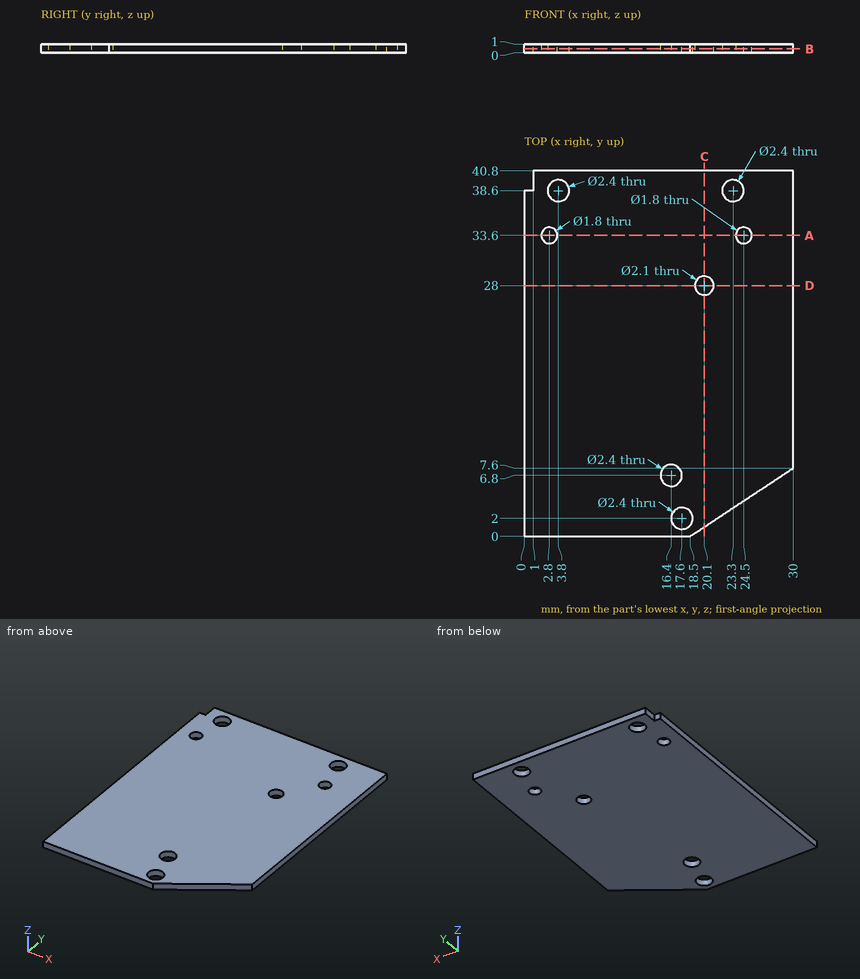
Source: three-view drawing plus pictorial views. Frame: mm from the lowest corner of the part. Coordinates: 2 decimals unless noted, no trailing zeros. Order: outer loops, then holes, each group sorted by start corner. A loop starts at its lowest first (then second) coordinate and runs counter-clockwise, first axis right, second up.
1) Section B-B (z = 0.45). Return loops of the section in (x, y), then the cut area to 3 significant figures.
Result sheet:
outline: (0, 0) - (18.5, 0) - (30, 7.6) - (30, 40.8) - (1, 40.8) - (1, 38.6) - (0, 38.6) - close; hole circle Ø1.8 at (2.8, 33.6); hole circle Ø2.4 at (3.8, 38.6); hole circle Ø2.4 at (16.4, 6.8); hole circle Ø2.4 at (17.6, 2); hole circle Ø2.1 at (20.1, 28); hole circle Ø2.4 at (23.3, 38.6); hole circle Ø1.8 at (24.5, 33.6)
area: 1,150 mm2
2) Section D-D (y = 28). Return loops of the section in (x, z).
Result sheet:
outline: (0, 0) - (19.05, 0) - (19.05, 1) - (0, 1) - close; (21.15, 0) - (30, 0) - (30, 1) - (21.15, 1) - close
3) Section A-A (y = 33.6). Return loops of the section in (x, z), then the cut area to 3 significant figures.
Result sheet:
outline: (0, 0) - (1.9, 0) - (1.9, 1) - (0, 1) - close; (3.7, 0) - (23.6, 0) - (23.6, 1) - (3.7, 1) - close; (25.4, 0) - (30, 0) - (30, 1) - (25.4, 1) - close
area: 26.4 mm2
4) Section C-C (x = 20.1). Return loops of the section in (y, z).
Result sheet:
outline: (1.06, 0) - (26.95, 0) - (26.95, 1) - (1.06, 1) - close; (29.05, 0) - (40.8, 0) - (40.8, 1) - (29.05, 1) - close
5) Ray query, probe 1 along X at (y, z) = (33.6, 0.65); probe 2 along X at (y, z) = (38.5, 0.3); probe 3 along Y at (x, z) = (2.75, 0.6). Return the intervals inside material, ascending.
Result sheet:
probe 1: x = 0 to 1.9, 3.7 to 23.6, 25.4 to 30
probe 2: x = 0 to 2.6, 5 to 22.1, 24.5 to 30
probe 3: y = 0 to 32.7, 34.5 to 38.02, 39.18 to 40.8
